Input: part model. Units: mm. Frame: model coordinates. A direction names the side the tool comes from. Give positions to 0.01 mm unless a question says otherwise; leave off trailing zeros. Order: outer loops, then holes, each group sorted by start corner. A loop starts at its lowest first (then second) coordinate and runs counter-clockwise, first axis right, second up. Notation, with made-up numbers: (-33, 17.5) - (3, 17.5) arc R16 cw to (3, 36.5) - close; hole circle Ø4 at (82, 38). An arc over 180 degrees is marked (long way). Use a Markdown table: item, result.
from build123d import *

# Parameters (mm, degrees)
SKETCH1_R           = 2
BOSS_EXTRUDE3_DEPTH = 9
SKETCH2_R           = 10.25
CUT_EXTRUDE1_DEPTH  = 6


with BuildPart() as part:
    # Sketch1 → Boss-Extrude3 (new body)
    # profile 1 of 5: a face of its own
    with BuildSketch(Plane.XY):
        with BuildLine():
            Line((-25, 8.5), (-25, -8.5))
            Line((-25, -8.5), (-15.297058541, -8.5))
            ThreePointArc((-15.297058541, -8.5), (-17.5, 0), (-15.297058541, 8.5))
            Line((-15.297058541, 8.5), (-25, 8.5))
        make_face()
        with Locations((-21, 0)):
            Circle(SKETCH1_R, mode=Mode.SUBTRACT)
    # profile 2 of 5: a face of its own
    with BuildSketch(Plane.XY):
        with BuildLine():
            ThreePointArc((15.297058541, 8.5), (0, 17.5), (-15.297058541, 8.5))
            Line((-15.297058541, 8.5), (15.297058541, 8.5))
        make_face()
    # profile 3 of 5: a face of its own
    with BuildSketch(Plane.XY):
        with BuildLine():
            ThreePointArc((-15.297058541, 8.5), (-17.5, 0), (-15.297058541, -8.5))
            Line((-15.297058541, -8.5), (15.297058541, -8.5))
            ThreePointArc((15.297058541, -8.5), (16.940314703, -4.390414305), (17.5, 0))
            ThreePointArc((17.5, 0), (16.940314703, 4.390414305), (15.297058541, 8.5))
            Line((15.297058541, 8.5), (-15.297058541, 8.5))
        make_face()
    # profile 4 of 5: a face of its own
    with BuildSketch(Plane.XY):
        with BuildLine():
            Line((15.297058541, -8.5), (-15.297058541, -8.5))
            ThreePointArc((-15.297058541, -8.5), (0, -17.5), (15.297058541, -8.5))
        make_face()
    # profile 5 of 5: a face of its own
    with BuildSketch(Plane.XY):
        with BuildLine():
            ThreePointArc((17.5, 0), (16.940314703, -4.390414305), (15.297058541, -8.5))
            Line((15.297058541, -8.5), (25, -8.5))
            Line((25, -8.5), (25, 8.5))
            Line((25, 8.5), (15.297058541, 8.5))
            ThreePointArc((15.297058541, 8.5), (16.940314703, 4.390414305), (17.5, 0))
        make_face()
        with Locations((21, 0)):
            Circle(SKETCH1_R, mode=Mode.SUBTRACT)
    extrude(amount=BOSS_EXTRUDE3_DEPTH)

    # Sketch2 → Cut-Extrude1 (cut)
    with BuildSketch(Plane.XY.offset(9)):
        Circle(SKETCH2_R)
    extrude(amount=-CUT_EXTRUDE1_DEPTH, mode=Mode.SUBTRACT)


solid = part.part
1. Pin query (flat end, axial travel): pin 1 (1.5 mm diameter, centred on x = -12, z = 2.5, fed in from +Y); pin 2 (4.5 mm diameter, centred on x = -20.5, z = 4.5, fed in from +Y); pin 3 (1 mm diameter, centred on x = -9.5, z = 5, fed in from +Y); pin 4 (3.5 mm diameter, centred on x = -21, y = 0, fed in from -Z). Return the tip coordinate at first contact, or that it passes through.
Response:
| item | result |
|---|---|
| pin 1 | stops at y = 13.4 |
| pin 2 | stops at y = 8.5 |
| pin 3 | stops at y = 15.01 |
| pin 4 | passes through |
2. Section query D-D (x = 0). Return loops of the section in (y, z), then the cut area to 3 significant figures.
Response:
| item | result |
|---|---|
| outline | (-17.5, 0) - (17.5, 0) - (17.5, 9) - (10.25, 9) - (10.25, 3) - (-10.25, 3) - (-10.25, 9) - (-17.5, 9) - close |
| area | 192 mm^2 |
3. Material intervals for line 1 along Y through (x, z) = (-21, 4.5); line 2 along Y through (x, z) = (4, 8.5); line 3 along Z through (x, y) = (-4.5, -7), sorted ascending.
Response:
| item | result |
|---|---|
| line 1 | y = -8.5 to -2, 2 to 8.5 |
| line 2 | y = -17.04 to -9.44, 9.44 to 17.04 |
| line 3 | z = 0 to 3 |
4. Section query A-A (y = 0). Return loops of the section in (x, z), then the cut area to 3 significant figures.
Response:
| item | result |
|---|---|
| outline | (-25, 0) - (-23, 0) - (-23, 9) - (-25, 9) - close; (-19, 0) - (19, 0) - (19, 9) - (10.25, 9) - (10.25, 3) - (-10.25, 3) - (-10.25, 9) - (-19, 9) - close; (23, 0) - (25, 0) - (25, 9) - (23, 9) - close |
| area | 255 mm^2 |
5. Set-up query: faces 4 (the face through (20, -8.5, 4)), 5 (the face through (20, 8.5, 4)), 6 (the face through (-20, 8.5, 4)), 7 (the face through (-2.222, -10.006, 6.042)), 8 (the face through (-20, -8.5, 4)). Return all of +Z, -Z, +X, -X, +Y, -Y with unobstructed straight access to the full face (end or side cutting, diameter ignored); none if empty.
Response:
| item | result |
|---|---|
| face 4 | +Z, -Z, +X, -Y |
| face 5 | +Z, -Z, +X, +Y |
| face 6 | +Z, -Z, -X, +Y |
| face 7 | +Z |
| face 8 | +Z, -Z, -X, -Y |
6. Section query B-B (x = 21). Return loops of the section in (y, z).
Response:
| item | result |
|---|---|
| outline | (-8.5, 0) - (-2, 0) - (-2, 9) - (-8.5, 9) - close; (2, 0) - (8.5, 0) - (8.5, 9) - (2, 9) - close |
7. Section query C-C (z = 4.5). Return loops of the section in (x, y).
Response:
| item | result |
|---|---|
| outline | (-25, -8.5) - (-15.3, -8.5) arc R17.5 ccw to (15.3, -8.5) - (25, -8.5) - (25, 8.5) - (15.3, 8.5) arc R17.5 ccw to (-15.3, 8.5) - (-25, 8.5) - close; hole circle Ø4 at (-21, 0); hole circle Ø20.5 at (0, 0); hole circle Ø4 at (21, 0) |
8. Mould query, pull axis X, two halves, no side actions, for faces 1 (the face through (0, 0, 3)), 2 (the face through (0.26, 17.5, 4.44)), 3 (the face through (-11, 0, 9)). Classes: pulls with the +X half, pulls with the -X half, needs draft (parallel to the pull), parting line crosses it, or undercut.
Response:
| item | result |
|---|---|
| face 1 | undercut |
| face 2 | parting line crosses it |
| face 3 | needs draft |
